Check sheet for the modelled part. Datum: model origin and axes. Units: mm. Face numbers are marked on the shaded views. A direction names the side the tool comes from. Coordinates: 2 decimals unless noted, no trailing zeros. Loops run counter-clockwise (first coordinate to the right, second up) from the corner with the lowest first, then second, coordinate; pieces in that order, holes last.
```python
from build123d import *

# Parameters (mm, degrees)
SKETCH1_W           = 20
SKETCH1_H           = 38
BOSS_EXTRUDE1_DEPTH = 40
SKETCH2_W           = 7
SKETCH2_H           = 2.5
BOSS_EXTRUDE2_DEPTH = 20
CUT_EXTRUDE1_DEPTH  = 40
SKETCH4_R           = 1.8
CUT_EXTRUDE2_DEPTH  = 10
SKETCH5_W           = 20
SKETCH5_H           = 40
CUT_EXTRUDE3_DEPTH  = 2
SKETCH6_R           = 6.75
SKETCH6_R_2         = 5.5
BOSS_EXTRUDE3_DEPTH = 0.5
SKETCH6_4_R         = 5.5
SKETCH6_4_R_2       = 3
BOSS_EXTRUDE4_DEPTH = 1.5
SKETCH6_5_R         = 3
BOSS_EXTRUDE5_DEPTH = 5


with BuildPart() as part:
    # Sketch1 → Boss-Extrude1 (new body)
    with BuildSketch(Plane.XY):
        with Locations((10, 19)):
            Rectangle(SKETCH1_W, SKETCH1_H)
    extrude(amount=BOSS_EXTRUDE1_DEPTH)

    # Sketch2 → Boss-Extrude2 (add)
    with BuildSketch(Plane.ZY):
        with Locations((-3.5, 28.25)):
            Rectangle(SKETCH2_W, SKETCH2_H)
        with Locations((43.5, 28.25)):
            Rectangle(SKETCH2_W, SKETCH2_H)
    extrude(amount=-BOSS_EXTRUDE2_DEPTH)

    # Sketch3 → Cut-Extrude1 (cut)
    with BuildSketch(Plane.ZY):
        Polygon((6, 38), (4, 36.5), (0, 36.5), (0, 38), align=None)
    extrude(amount=-CUT_EXTRUDE1_DEPTH, mode=Mode.SUBTRACT)

    # Sketch4 → Cut-Extrude2 (cut)
    with BuildSketch(Plane(origin=(0, 29.5, 0), x_dir=(1, 0, 0), z_dir=(0, 1, 0))):
        with Locations((15, -44.7)):
            Circle(SKETCH4_R)
        with Locations((5, -44.7)):
            Circle(SKETCH4_R)
        with Locations((15, 4.7)):
            Circle(SKETCH4_R)
        with Locations((5, 4.7)):
            Circle(SKETCH4_R)
    extrude(amount=-CUT_EXTRUDE2_DEPTH, mode=Mode.SUBTRACT)

    # Sketch5 → Cut-Extrude3 (cut)
    with BuildSketch(Plane(origin=(0, 38, 0), x_dir=(1, 0, 0), z_dir=(0, 1, 0))):
        with Locations((10, -20)):
            Rectangle(SKETCH5_W, SKETCH5_H)
        with BuildLine():
            Line((19.449743203, -29.975974241), (19.449743203, -0.575747889))
            Line((19.449743203, -0.575747889), (0.449743203, -0.575747889))
            Line((0.449743203, -0.575747889), (0.449743203, -29.975974241))
            ThreePointArc((0.449743203, -29.975974241), (9.949743203, -39.475974241), (19.449743203, -29.975974241))
        make_face(mode=Mode.SUBTRACT)
    extrude(amount=-CUT_EXTRUDE3_DEPTH, mode=Mode.SUBTRACT)

    # Sketch6 → Boss-Extrude3 (add)
    with BuildSketch(Plane(origin=(0, 38, 0), x_dir=(1, 0, 0), z_dir=(0, 1, 0))):
        with Locations((10, -30)):
            Circle(SKETCH6_R)
        with Locations((10, -30)):
            Circle(SKETCH6_R_2, mode=Mode.SUBTRACT)
    extrude(amount=BOSS_EXTRUDE3_DEPTH)

    # Sketch6<4> → Boss-Extrude4 (add)
    with BuildSketch(Plane(origin=(0, 38, 0), x_dir=(1, 0, 0), z_dir=(0, 1, 0))):
        with Locations((10, -30)):
            Circle(SKETCH6_4_R)
        with Locations((10, -30)):
            Circle(SKETCH6_4_R_2, mode=Mode.SUBTRACT)
    extrude(amount=BOSS_EXTRUDE4_DEPTH)

    # Sketch6<5> → Boss-Extrude5 (add)
    with BuildSketch(Plane(origin=(0, 38, 0), x_dir=(1, 0, 0), z_dir=(0, 1, 0))):
        with Locations((10, -30)):
            Circle(SKETCH6_5_R)
    extrude(amount=BOSS_EXTRUDE5_DEPTH)


solid = part.part
```
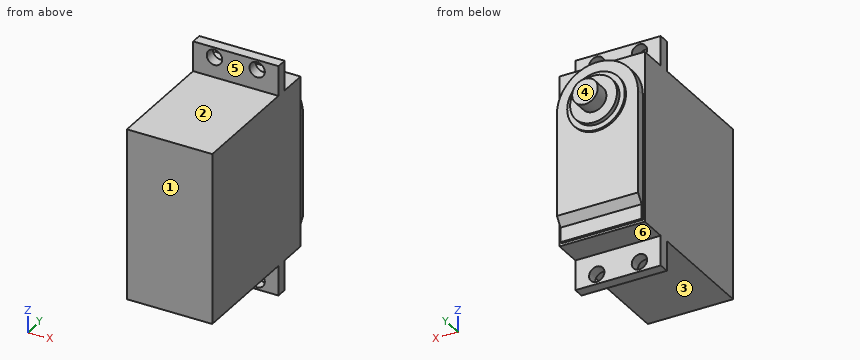
1) Depth check by flat-ended pin: pin 1 (6 mm diameter, centred on x = 5, z = 44.7, fed in from +Y); pin 2 (10 mm diameter, centred on x = 13, z = 14.5, fed in from +Y); pin 3 (12 mm diameter, centred on x = 16, y = 16, fed in from +Z). Enter the tip coordinate at first touch or a pass-through.
Answer sheet:
pin 1: stops at y = 29.5
pin 2: stops at y = 38
pin 3: stops at z = 40
2) Section check D-D on x = 1.5. Enter the section's corners in (y, z), plus the area to 3 significant figures.
Answer sheet:
outline: (0, 0) - (27, 0) - (27, -7) - (29.5, -7) - (29.5, 0) - (36, 0) - (36, 0.58) - (36.5, 0.58) - (36.5, 4) - (38, 6) - (38, 34.32) - (36, 34.32) - (36, 40) - (29.5, 40) - (29.5, 47) - (27, 47) - (27, 40) - (0, 40) - close
area: 1,540 mm2
3) Set-up check for the marked faces 4, 5 and 6: record each of +Z, -Z, +X, -X, +Y, -Y from which the full face is reachable in a straight line by a thin tool's end or side.
Answer sheet:
face 4: +Z, -Z, +X, -X, +Y
face 5: +Z, +X, -X, -Y
face 6: -Z, +X, -X, +Y
4) Scan lines: line 1 (X direction, y = 28.9, z = -4.7); line 2 (Z direction, x = 5, y = 28.15); line 3 (Z direction, x = 18.25, y = 18). Record each from-to range of solid material in increasing order.
Answer sheet:
line 1: x = 0 to 3.2, 6.8 to 13.2, 16.8 to 20
line 2: z = -7 to -6.5, -2.9 to 42.9, 46.5 to 47
line 3: z = 0 to 40
5) Section check A-A on z = 44.7. Enter the section's corners in (x, y), plus the area to 3 significant figures.
Answer sheet:
outline: (0, 27) - (3.2, 27) - (3.2, 29.5) - (0, 29.5) - close; (6.8, 27) - (13.2, 27) - (13.2, 29.5) - (6.8, 29.5) - close; (16.8, 27) - (20, 27) - (20, 29.5) - (16.8, 29.5) - close
area: 32.0 mm2
6) Section check C-C on z = 7.5. Enter the section's corners in (x, y).
Answer sheet:
outline: (0, 0) - (20, 0) - (20, 36) - (19.45, 36) - (19.45, 38) - (0.45, 38) - (0.45, 36) - (0, 36) - close
7) Mould release check, pull along Z, two halves, no side actions. Record for the marked faces 1, 2 and 3: +Z half, -Z half, draft (parallel to the pull), parting line (faces both ways), or undercut.
Answer sheet:
face 1: draft
face 2: +Z half
face 3: -Z half
8) Section check B-B on x = 14.75. Give the number of separate pieces and of enclosed holes in the cut face, plus the area to 3 significant figures.
Answer sheet:
separate pieces: 3
enclosed holes: 0
area: 1,540 mm2
